```python
from build123d import *

# Parameters (mm, degrees)
SKIZZE1_W                           = 70
SKIZZE1_H                           = 28
AUFSATZ_LINEAR_AUSTRAGEN1_DEPTH     = 4
SKIZZE2_R                           = 2.15
AUFSATZ_LINEAR_AUSTRAGEN2_DEPTH     = 6
VERRUNDUNG1_R                       = 6.5
VERRUNDUNG1_OF_SPIEGELN1_R          = 6.5
FASE1_SIZE                          = 4
VERRUNDUNG2_R                       = 2
SCHNITT_LINEAR_START                = -5
SCHNITT_LINEAR_AUSTRAGEN1_OUTLINE_W = 6.179640558
SCHNITT_LINEAR_AUSTRAGEN1_OUTLINE_H = 16
SCHNITT_LINEAR_AUSTRAGEN1_DEPTH     = 5.828427125
SCHNITT_LINEAR_AUSTRAGEN2_REACH     = 40.756
SKIZZE4_R                           = 1.25
FASE2_SIZE                          = 0.5


with BuildPart() as part:
    # Skizze1 → Aufsatz-Linear austragen1 (new body)
    with BuildSketch(Plane(origin=(0, 0, 0), x_dir=(1, 0, 0), z_dir=(0, 1, 0))):
        Rectangle(SKIZZE1_W, SKIZZE1_H)
    extrude(amount=AUFSATZ_LINEAR_AUSTRAGEN1_DEPTH)

    # Skizze2 → Aufsatz-Linear austragen2 (add)
    with BuildSketch(Plane.XY.offset(14)):
        Polygon((16.807611845, 4), (25.807611845, 13), (35, 13), (35, 4), align=None)
        with Locations((28.5, 6.5)):
            Circle(SKIZZE2_R, mode=Mode.SUBTRACT)
    aufsatz_linear_austragen2 = extrude(amount=-AUFSATZ_LINEAR_AUSTRAGEN2_DEPTH)

    # Verrundung1
    verrundung1_edges = [part.edges().sort_by_distance(p)[0] for p in [
        (25.807611845, 13, 11),
        (35, 13, 11),
    ]]
    fillet(verrundung1_edges, radius=VERRUNDUNG1_R - 0.0001)  # a hair under: the kernel refuses the full size

    # Spiegeln1: Aufsatz-Linear austragen2 across plane
    add(aufsatz_linear_austragen2.mirror(Plane.XY))

    # Verrundung1 of Spiegeln1
    verrundung1_of_spiegeln1_edges = [part.edges().sort_by_distance(p)[0] for p in [
        (25.807611845, 13, -11),
        (35, 13, -11),
    ]]
    fillet(verrundung1_of_spiegeln1_edges, radius=VERRUNDUNG1_OF_SPIEGELN1_R - 0.0001)  # a hair under: the kernel refuses the full size

    # Fase1
    fase1_edges = [part.edges().sort_by_distance(p)[0] for p in [
        (35, 0, 0),
    ]]
    chamfer(fase1_edges, length=FASE1_SIZE - 0.0001)  # a hair under: the kernel refuses the full size

    # Verrundung2
    # the kernel refuses this fillet: 2 mm, written as the material it takes off along each edge
    with BuildSketch(Plane(origin=(31.0001, 0, 16.071067812), x_dir=(0.7071067811865477, 0.7071067811865474, 0), z_dir=(0, 0, -1)), Plane(origin=(35, 3.9999, 16.071067812), x_dir=(0, 1, 0), z_dir=(0, 0, -1))) as verrundung2_piece_1:
        with BuildLine():
            CenterArc((VERRUNDUNG2_R * 0.414213562373, -VERRUNDUNG2_R), VERRUNDUNG2_R, 90, 45)
            Line((-VERRUNDUNG2_R * 0.292893218813, -VERRUNDUNG2_R * 0.292893218813), (0, 0))
            Line((0, 0), (VERRUNDUNG2_R * 0.414213562373, 0))
        make_face()
    extrude(amount=32.142135624, mode=Mode.SUBTRACT)

    # Schnitt-Linear austragen1: read off the stored shape, not the designer's step
    # Schnitt-Linear austragen1 outline → Schnitt-Linear austragen1 (cut)
    with BuildSketch(Plane(origin=(0, 4, 0), x_dir=(1, 0, 0), z_dir=(0, 1, 0)).offset(SCHNITT_LINEAR_START)):
        with Locations((32.910179721, 0)):
            Rectangle(SCHNITT_LINEAR_AUSTRAGEN1_OUTLINE_W, SCHNITT_LINEAR_AUSTRAGEN1_OUTLINE_H)
    extrude(amount=SCHNITT_LINEAR_AUSTRAGEN1_DEPTH, mode=Mode.SUBTRACT)

    # Skizze4 → Schnitt-Linear austragen2 (cut, up to next)
    with BuildSketch(Plane(origin=(0, 4, 0), x_dir=(1, 0, 0), z_dir=(0, 1, 0)), mode=Mode.PRIVATE) as schnitt_linear_austragen2_sk1:
        with Locations(Location((-19.1, -10.85, 0), (0, 0, 270))):
            Circle(SKIZZE4_R)
    schnitt_linear_austragen2_tool1 = extrude(schnitt_linear_austragen2_sk1.sketch, amount=-SCHNITT_LINEAR_AUSTRAGEN2_REACH, mode=Mode.PRIVATE) & part.part
    # Skizze4 → Schnitt-Linear austragen2 (cut, up to next)
    with BuildSketch(Plane(origin=(0, 4, 0), x_dir=(1, 0, 0), z_dir=(0, 1, 0)), mode=Mode.PRIVATE) as schnitt_linear_austragen2_sk2:
        with Locations(Location((9.4, 0, 0), (0, 0, 270))):
            Circle(SKIZZE4_R)
    schnitt_linear_austragen2_tool2 = extrude(schnitt_linear_austragen2_sk2.sketch, amount=-SCHNITT_LINEAR_AUSTRAGEN2_REACH, mode=Mode.PRIVATE) & part.part
    # Skizze4 → Schnitt-Linear austragen2 (cut, up to next)
    with BuildSketch(Plane(origin=(0, 4, 0), x_dir=(1, 0, 0), z_dir=(0, 1, 0)), mode=Mode.PRIVATE) as schnitt_linear_austragen2_sk3:
        with Locations(Location((-19.1, 10.85, 0), (0, 0, 270))):
            Circle(SKIZZE4_R)
    schnitt_linear_austragen2_tool3 = extrude(schnitt_linear_austragen2_sk3.sketch, amount=-SCHNITT_LINEAR_AUSTRAGEN2_REACH, mode=Mode.PRIVATE) & part.part
    add(schnitt_linear_austragen2_tool1.solids().sort_by_distance((-19.1, 4, 10.85))[0], mode=Mode.SUBTRACT)
    add(schnitt_linear_austragen2_tool2.solids().sort_by_distance((9.4, 4, 0))[0], mode=Mode.SUBTRACT)
    add(schnitt_linear_austragen2_tool3.solids().sort_by_distance((-19.1, 4, -10.85))[0], mode=Mode.SUBTRACT)

    # Fase2
    # the kernel refuses this chamfer: 0.5 mm, written as the material it takes off along each edge
    with BuildSketch(Plane(origin=(-36.285841494, 0, 14), x_dir=(0, 0, -1), z_dir=(1, 0, 0))) as fase2_piece_1:
        Polygon((FASE2_SIZE, 0), (0, FASE2_SIZE), (0, 0), align=None)
    extrude(amount=68.643444909, mode=Mode.SUBTRACT)
    with BuildSketch(Plane(origin=(-35, 0, -15.285841494), x_dir=(1, 0, 0), z_dir=(0, 0, 1))) as fase2_piece_2:
        Polygon((FASE2_SIZE, 0), (0, FASE2_SIZE), (0, 0), align=None)
    extrude(amount=30.571682988, mode=Mode.SUBTRACT)
    with BuildSketch(Plane(origin=(32.357603415, 0, -14), x_dir=(0, 1, 0), z_dir=(-1, 0, 0))) as fase2_piece_3:
        Polygon((FASE2_SIZE, 0), (0, -FASE2_SIZE), (0, 0), align=None)
    extrude(amount=68.643444909, mode=Mode.SUBTRACT)
    with BuildSketch(Plane(origin=(29.820359442, 0, 8), x_dir=(-1, 0, 0), z_dir=(0, 0, -1))) as fase2_piece_4:
        Polygon((FASE2_SIZE, 0), (0, FASE2_SIZE), (0, 0), align=None)
    extrude(amount=16, mode=Mode.SUBTRACT)


solid = part.part
```
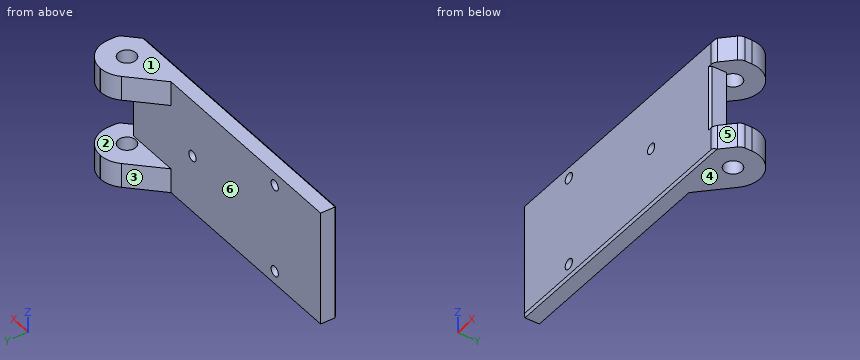
For this review, take the finished solid that the model builds, in its own axes (mm). Face numbers are marked on the shaded views. A direction names the side the tool comes from. Round coordinates to 2 decimals unless told otherwise and drop trailing zeros. Loops run counter-clockwise (first coordinate to the right, second up) from the corner with the lowest first, then second, coordinate; pieces in that order, holes last.
(1) We need section D-D (z = 0.5). Give the boundary of the cut face in (x, y), plus the area to 3 significant figures.
Returned:
outline: (-35, 0.5) - (-34.5, 0) - (8.25, 0) - (8.25, 4) - (-35, 4) - close; (10.55, 0) - (29.32, 0) - (29.82, 0.5) - (29.82, 4) - (10.55, 4) - close
area: 250 mm2
(2) Wall thickness on line 1 along X through (y, z) = (1.75, 0); line 2 along Y through (x, z) = (28.5, -9.2); line 3 along Y through (x, z) = (-7, -12.5): over which ranges is each line inside the solid? List them lowest first.
Returned:
line 1: x = -35 to 8.15, 10.65 to 29.82
line 2: y = 0 to 4.35, 8.65 to 13
line 3: y = 0 to 4
(3) We need section B-B (x = -19.1). Give the boundary of the cut face in (y, z), plus the area to 4 significant figures.
Returned:
outline: (0, -13.5) - (0.5, -14) - (4, -14) - (4, -12.1) - (0, -12.1) - close; (0, -9.6) - (4, -9.6) - (4, 9.6) - (0, 9.6) - close; (0, 12.1) - (4, 12.1) - (4, 14) - (0.5, 14) - (0, 13.5) - close
area: 91.75 mm2
(4) Tool access review of the marked faces 5 and 6: name each direction out of +Z, -Z, +X, -X, +Y, -Y from which nothing blocks a thin tool from reaching the whole face with its end or side.
Returned:
face 5: +Z, -Z, +X, -Y
face 6: -X, +Y
(5) We need section A-A (z = -10.85). State how many separate pieces and enclosed holes the cut face has, plus the area to 3 significant figures.
Returned:
separate pieces: 2
enclosed holes: 1
area: 360 mm2
(6) Mouldability with a two-part tool opening along Z and no side actions: class the marked faces 1, 2, 3 and 4 as released by +Z, released by -Z, zero draft, split by the parting line, or undercut.
Returned:
face 1: released by +Z
face 2: undercut
face 3: zero draft
face 4: released by -Z
(7) Clearance check with flat-ended pins moving along their axes: P1, Ø3, axis at x = 9.4, z = 0, coming from the +Y side; P2, Ø1.5, axis at x = -19.1, z = 10.85, coming from the +Y side; P3, Ø4, axis at y = 1.5, z = 1.5, coming from the +X side. State where each tip first meets the part, or that it passes through.
Returned:
P1: stops at y = 4
P2: passes through
P3: stops at x = 29.82
(8) We need section C-C (x = 9.4). Give the boundary of the cut face in (y, z).
Returned:
outline: (0, -13.5) - (0.5, -14) - (4, -14) - (4, -1.25) - (0, -1.25) - close; (0, 1.25) - (4, 1.25) - (4, 14) - (0.5, 14) - (0, 13.5) - close
